Autodesk Inventor part; units mm, degrees
ref_plane "YZ Plane" through (0, 0, 0) normal (1, 0, 0) x (0, 1, 0)
ref_plane "XZ Plane" through (0, 0, 0) normal (0, 1, 0) x (-1, 0, 0)
ref_plane "XY Plane" through (0, 0, 0) normal (0, 0, 1) x (1, 0, 0)
ref_plane "Work Plane1" through (0, 0, 0) normal (0, 0, 1) x (1, 0, 0)
sketch "Sketch1" plane through (0, 0, 0) normal (0, 0, 1) x (1, 0, 0)
  line L0 (250, 0) -> (0, 0) construction
  line L1 (250, 0) -> (250, 20) construction
  line L2 (0, 20) -> (250, 20) construction
  line L3 (0, 0) -> (0, 20) construction
  line L4 (245, 20) -> (153.1686, 20) construction
  line L5 (245, 20) -> (245, 80) construction
  line L6 (153.1686, 80) -> (245, 80) construction
  line L7 (153.1686, 20) -> (153.1686, 80) construction
  line L8 (-5, 0) -> (255, 0)
  line L9 (255, 0) -> (255, 70)
  line L10 (255, 70) -> (230, 70)
  line L11 (230, 70) -> (230, 65)
  line L12 (230, 65) -> (20, 65)
  line L13 (20, 65) -> (20, 70)
  line L14 (20, 70) -> (-5, 70)
  line L15 (-5, 70) -> (-5, 0)
  dimension "d0" = 10
  dimension "d1" = 5
  dimension "d2" = 5
  dimension "d3" = 5
  dimension "d4" = 25
  dimension "d5" = 25
extrude "Extrusion1" add sketch "Sketch1" along normal blind 5
hole "Hole1" [suppressed]
hole "Hole2" [suppressed]
sketch "Sketch2" plane through (0, 0, 0) normal (0, 0, -1) x (-1, 0, 0)
  line L0 (0, 0) -> (-250, 0) construction
  line L1 (0, 0) -> (0, 20) construction
  line L2 (-250, 20) -> (0, 20) construction
  line L3 (-250, 0) -> (-250, 20) construction
  line L4 (5, 0) -> (-255, 0) construction
  line L5 (5, 70) -> (5, 0) construction
  line L6 (-20, 70) -> (5, 70) construction
  line L7 (-20, 65) -> (-20, 70) construction
  line L8 (-230, 65) -> (-20, 65) construction
  line L9 (-230, 70) -> (-230, 65) construction
  line L10 (-255, 70) -> (-230, 70) construction
  line L11 (-255, 0) -> (-255, 70) construction
  line L12 (-125, 20) -> (-125, 0) construction
  line L13 (-250, 10) -> (0, 10) construction
  point P0 (-125, 10)
  point P1 (-230, 10)
  point P2 (-20, 10)
  dimension "d30" = 20
  dimension "d31" = 20
hole "Hole3" [suppressed]
sketch "Sketch3" plane through (20, 65, 0) normal (0, 1, 0) x (1, 0, 0)
  line L0 (210, 0) -> (0, 0) construction
  line L1 (0, 0) -> (0, -5) construction
  line L2 (210, -5) -> (0, -5) construction
  line L3 (210, 0) -> (210, -5) construction
  line L4 (210, 0) -> (210, -5) construction
  line L5 (0, 0) -> (0, -5) construction
  line L6 (0, -2.5) -> (210, -2.5) construction
  line L7 (-25, -5) -> (235, -5) construction
  line L8 (105, -5) -> (105, 0) construction
  line L9 (-25, 0) -> (235, 0) construction
  point P0 (-20, 0)
  point P1 (105, -2.5)
  point P2 (20, -2.5)
  point P3 (190, -2.5)
  dimension "d39" = 20
  dimension "d40" = 20
hole "Hole4" at (125, 65, 2.5) at (40, 65, 2.5) at (210, 65, 2.5) direction (0, -1, 0) diameter 2.459 depth 8.8 tip angle 118
sketch "Sketch4" plane through (0, 0, 5) normal (0, 0, 1) x (1, 0, 0)
  line L0 (41.2295, 56.2) -> (41.2295, 65) construction
  line L1 (38.7705, 56.2) -> (38.7705, 65) construction
  line L2 (126.2295, 56.2) -> (126.2295, 65) construction
  line L3 (123.7705, 56.2) -> (123.7705, 65) construction
  line L4 (208.7705, 56.2) -> (208.7705, 65) construction
  line L5 (211.2295, 56.2) -> (211.2295, 65) construction
  line L6 (37.15, 62) -> (42.85, 62)
  line L7 (42.85, 62) -> (42.85, 59)
  line L8 (42.85, 59) -> (37.15, 59)
  line L9 (37.15, 59) -> (37.15, 62)
  line L10 (38.7705, 65) -> (41.2295, 65) construction
  line L11 (230, 65) -> (20, 65) construction
  line L12 (40, 65) -> (40, 60.5) construction
  line L13 (122.15, 62) -> (127.85, 62)
  line L14 (127.85, 62) -> (127.85, 59)
  line L15 (127.85, 59) -> (122.15, 59)
  line L16 (122.15, 59) -> (122.15, 62)
  line L17 (123.7705, 65) -> (126.2295, 65) construction
  line L18 (125, 65) -> (125, 61.2984) construction
  line L19 (212.85, 62) -> (212.85, 59)
  line L20 (210, 65) -> (210, 58.9) construction
  line L21 (208.7705, 65) -> (211.2295, 65) construction
  line L22 (207.15, 62) -> (212.85, 62)
  line L23 (212.85, 59) -> (207.15, 59)
  line L24 (207.15, 59) -> (207.15, 62)
  point P0 (0, 0)
  dimension "d48" = 3
  dimension "d50" = 5.7
  dimension "d51" = 3
  dimension "d52" = 3
  dimension "d53" = 5.7
  dimension "d54" = 3
  dimension "d55" = 3
  dimension "d56" = 5.7
  dimension "d57" = 3
extrude "Extrusion2" cut sketch "Sketch4" against normal through all
sketch "Sketch5" plane through (0, 0, 5) normal (0, 0, 1) x (1, 0, 0)
  arc A0 (63, 35) -> (55, 35) centre (59, 35) ccw
  line L0 (63, 35) -> (63, 0)
  line L1 (55, 0) -> (55, 35)
  line L2 (55, 0) -> (63, 0)
  line L3 (-5, 0) -> (255, 0)
  point P0 (0, 0)
extrude "Extrusion3" [suppressed]
equation "\"d1\" = ABS_tolerance + plate_thickness"
equation "\"d2\" = plate_thickness + basic_plate_offset"
equation "\"d3\" = plate_thickness + basic_plate_offset"
equation "\"d5\" = d4"
equation "\"d6\" = plate_thickness"
equation "\"d52\" = d48"
equation "\"d53\" = d50"
equation "\"d55\" = d58"
equation "\"d56\" = d59"
equation "\"plate_thickness\" = 5"
equation "\"ABS_tolerance\" = 0"
equation "\"laser_cutter_thickness\" = 0.1"
equation "\"basic_plate_offser\" = 0.5"
equation "\"basic_plate_offset\" = 0"
properties part number "sides-02"
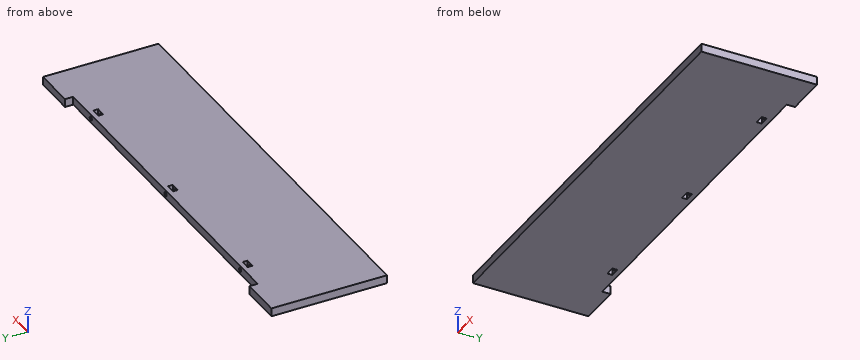
Can you work these out from the model? Positions are in its coordinate system, mm. Give positions to 0.01 mm unless a question says otherwise; leave off trailing zeros. Order: outer loops, then holes, each group sorted by start corner. A loop starts at its lowest first (then second) coordinate and runs counter-clockwise, first axis right, second up. Notation, with made-up numbers: M 26.25,69.25 L 54.25,69.25 A4 cw 54.25,74.25 Z; hole C -29.5,7 d2. An arc over 180 degrees is marked long. Use a Markdown table: item, result. Add a question column.
Item 1: Will these pins go through, and if not, where does the flat tip stop? pin 1 (2.5 mm diameter, centred on x = 210, z = 3.5, fed in from -Y); pin 2 (2 mm diameter, centred on x = 210, z = 2.5, fed in from +Y); pin 3 (1 mm diameter, centred on x = 90.5, z = 3.5, fed in from +Y); pin 4 (1.5 mm diameter, centred on x = 40, z = 2.5, fed in from +Y).
Item 2: Suppose I cut it at A-A (x = 179). List the corners of the cut face in (y, z) for me.
Item 3: If I drill on L1, parallel to X at y = 56.8, z = 2.5; L2, parallel to Z at x = 40, y = 64.2; L3, parallel to Y at x = 198.5, z = 0.6, over which ranges is the centre line in solid material (lowest first)? Write a range as [from, to].
Answer sheet:
| question | item | result |
|---|---|---|
| 1 | pin 1 | stops at y = 0 |
| 1 | pin 2 | stops at y = 56.06 |
| 1 | pin 3 | stops at y = 65 |
| 1 | pin 4 | stops at y = 55.91 |
| 2 | outline | M 0,0 L 65,0 L 65,5 L 0,5 Z |
| 3 | L1 | x = [-5, 38.77], [41.23, 123.77], [126.23, 208.77], [211.23, 255] |
| 3 | L2 | z = [0, 1.27], [3.73, 5] |
| 3 | L3 | y = [0, 65] |
